Geometry check sheet. Reference: drawing and pictorial views, mm from the part's lowest x, y, z. A direction names the side the tool comes from. Round coordinates to 2 decimals unless told otherwise and drop trailing zeros. Write each loop counter-clockwise with the first axis right and the second up, starting at its lowest first coordinate (ties: lowest second). Pieces come first, ordered by that corner, then holes. Notation, with made-up numbers: M 70,86 L 124,86 A23 cw 124,110 Z; hole C 0.25,-5.5 d1. An arc over 180 degrees is marked long. Put each result on its own line as item: value. Start each with the question number.
(1) Section check C-C on y = 8. Record the cut outline in (x, z).
(2) Tool access check on the marked faces 1 and 2. Record the directions out of +Z, -Z, +X, -X, +Y, -Y that give a thin tool (end or side, any length) a straight path to the whole face; none if there is none.
(3) Section check B-B on x = 5.5. Record the cut outline in (y, z).
(4) Gauge pin test, flat ends, axial feed: pin 1 (1.5 mm diameter, centred on x = 2.5, z = 5.5, fed in from +Y); pin 2 (2 mm diameter, centred on y = 1.5, z = 3.5, fed in from -X); pin 3 (5 mm diameter, centred on y = 5.5, z = 5.5, fed in from -X); pin 4 (2 mm diameter, centred on x = 10.5, y = 6, fed in from -Z). Record the tip position at first contact, or that the pin passes through.
(5) Section check D-D on y = 11.75. Record the cut outline in (x, z) (1 decimal), then the cut area to 3 significant figures.
(6) Material ranges on probe 1 along Y at (x, z) = (7, 7.5); probe 2 along Y at (x, z) = (10, 7.5) (1 decimal); probe 3 along X at (y, z) = (2.75, 10.5) (1 decimal), recorded low to high.
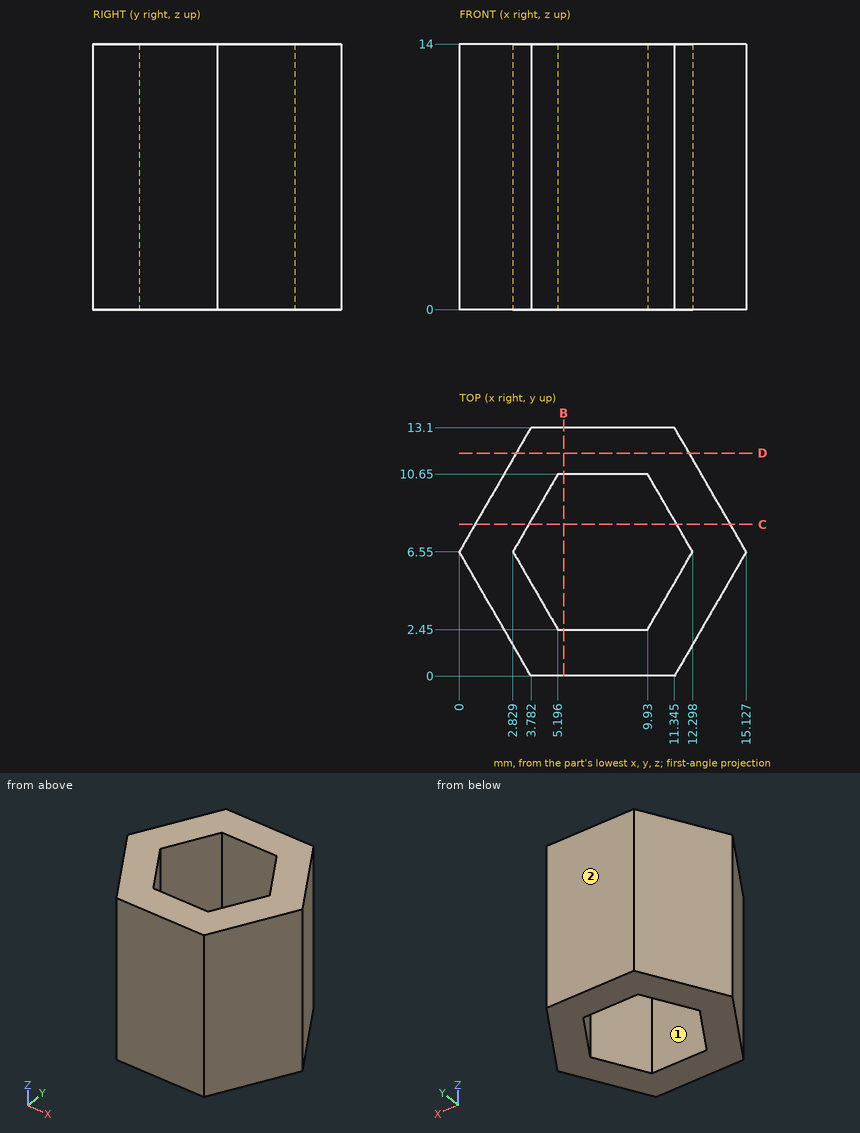
Answers follow:
1. outline: M 0.84,0 L 3.67,0 L 3.67,14 L 0.84,14 Z; M 11.46,0 L 14.29,0 L 14.29,14 L 11.46,14 Z
2. face 1: +Z, -Z
2. face 2: +Z, -Z, +X, -X, +Y
3. outline: M 0,0 L 2.45,0 L 2.45,14 L 0,14 Z; M 10.65,0 L 13.1,0 L 13.1,14 L 10.65,14 Z
4. pin 1: stops at y = 12.18
4. pin 2: stops at x = 2.34
4. pin 3: stops at x = 0
4. pin 4: passes through
5. outline: M 3,0 L 12.1,0 L 12.1,14 L 3,14 Z
5. area: 128 mm^2
6. probe 1: y = 0 to 2.45, 10.65 to 13.1
6. probe 2: y = 0 to 2.6, 10.5 to 13.1
6. probe 3: x = 2.2 to 5, 10.1 to 12.9
